Read the model definition and answer for the solid it produces. Units are mm, in the model's axes. Give positions to 0.01 mm unless a question says otherwise; leave off trailing zeros. Write each loop counter-clockwise with the first axis right and the second up, starting at its lowest first coordinate (ties: lowest second). Pieces come first, ordered by that corner, then holes.
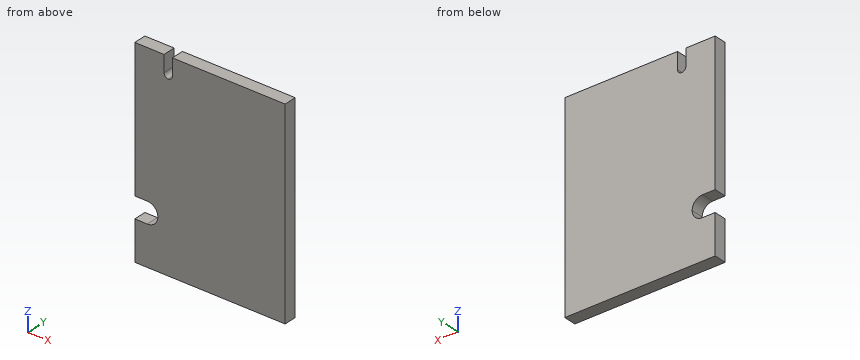
```python
from build123d import *

# Parameters (mm, degrees)
SKETCH1_W           = 228.6
SKETCH1_H           = 304.8
BOSS_EXTRUDE2_DEPTH = 19.05
CUT_EXTRUDE1_DEPTH  = 19.05


with BuildPart() as part:
    # Sketch1 → Boss-Extrude2 (new body)
    with BuildSketch(Plane(origin=(0, 0, 0), x_dir=(1, 0, 0), z_dir=(0, 1, 0))):
        with Locations((114.3, 152.4)):
            Rectangle(SKETCH1_W, SKETCH1_H)
    extrude(amount=BOSS_EXTRUDE2_DEPTH)

    # Sketch3 → Cut-Extrude1 (cut)
    with BuildSketch(Plane.XZ):
        with BuildLine():
            Line((19.125478143, -212.832325894), (0, -212.832325894))
            Line((0, -212.832325894), (0, -244.582325894))
            Line((0, -244.582325894), (19.125478143, -244.582325894))
            ThreePointArc((19.125478143, -244.582325894), (30.350798294, -239.932646046), (35.000478143, -228.707325894))
            ThreePointArc((35.000478143, -228.707325894), (30.350798294, -217.482005743), (19.125478143, -212.832325894))
        make_face()
        with BuildLine():
            Line((44.449497967, -25.319930082), (44.449497967, 0))
            Line((44.449497967, 0), (57.149497967, 0))
            Line((57.149497967, 0), (57.149497967, -25.319930082))
            ThreePointArc((57.149497967, -25.319930082), (55.289626028, -29.810058143), (50.799497967, -31.669930082))
            ThreePointArc((50.799497967, -31.669930082), (46.309369907, -29.810058143), (44.449497967, -25.319930082))
        make_face()
    extrude(amount=-CUT_EXTRUDE1_DEPTH, mode=Mode.SUBTRACT)


solid = part.part
```
Item 1: This flat-tipped pin is pushed along its axis until it touches: pin 1 Ø5 at (x, z) = (181, -97) entering from -Y. Where does it stop, or does it pass through?
Result set:
pin 1: stops at y = 0
Item 2: Find the intervals of material crossed by line 1 along Z through (x, y) = (18, 9.75); line 2 along X through (y, z) = (11.5, -22.5); line 3 along Z through (x, y) = (52, 15.5), in increasing order.
Result set:
line 1: z = -304.8 to -244.58, -212.83 to 0
line 2: x = 0 to 44.45, 57.15 to 228.6
line 3: z = -304.8 to -31.56
Item 3: Section A-A (x = 15) is taken. Write down the section's boundary in (y, z).
Result set:
outline: (0, -304.8) - (19.05, -304.8) - (19.05, -244.58) - (0, -244.58) - close; (0, -212.83) - (19.05, -212.83) - (19.05, 0) - (0, 0) - close
